Work out the finished part from the listing and answer in its coordinate system (mm). Coordinates: 2 decimals unless noted, no trailing zeros. Write each loop counter-clockwise with the first axis right and the second up, starting at its lowest first coordinate (ties: lowest second). Pieces come first, ordered by that corner, then holes. Notation, with made-up numbers: M 19.5,72.25 L 51.5,72.25 A17 ccw 51.5,88.25 Z; hole C 69.5,69 d10. An arc over 180 degrees is marked long. Answer as CSV lines item,"result". Start each with the question number.
(1) Find the intervals of material crossed by L1, parallel to X at y = 3.15, z = 10.5; L2, parallel to Z at x = 33, y = 2.45, in increasing order. Write a range as [from, to].
(2) A cutting plane is placed at A-A on z = 38.5. Give the vertices of the cut face in (x, y), then the cut area to 3 significant figures.
(3) The mould has two halves that part along X. Classify faces 1 (the flat face through (55, 0, 25)), 2 (the flat face through (78, 3, 27)), 3 (the flat face through (112, 3, 25)): released by +X, released by -X, zero draft, split by the parting line, or undercut.
(4) A cutting plane is placed at B-B on y = 1.25. Count the separate pieces of the cut face and the enclosed holes in it, then the cut area to 3 significant figures.
from build123d import *

# Parameters (mm, degrees)
SKETCH_1_W      = 112
SKETCH_1_H      = 50
SKETCH_1_W_2    = 3
SKETCH_1_H_2    = 20
SKETCH_1_W_3    = 3.2
EXTRUDE_1_DEPTH = 6


with BuildPart() as part:
    # 草图1 → 凸台-拉伸1 (new body)
    with BuildSketch(Plane(origin=(0, 0, 0), x_dir=(1, 0, 0), z_dir=(0, 1, 0))):
        with Locations((56, -25)):
            Rectangle(SKETCH_1_W, SKETCH_1_H)
        with Locations((4.5, -13)):
            Rectangle(SKETCH_1_W_2, SKETCH_1_H_2, mode=Mode.SUBTRACT)
        with Locations((4.5, -37)):
            Rectangle(SKETCH_1_W_2, SKETCH_1_H_2, mode=Mode.SUBTRACT)
        with Locations((107.5, -13)):
            Rectangle(SKETCH_1_W_2, SKETCH_1_H_2, mode=Mode.SUBTRACT)
        with Locations((107.5, -37)):
            Rectangle(SKETCH_1_W_2, SKETCH_1_H_2, mode=Mode.SUBTRACT)
        with Locations((34.4, -37)):
            Rectangle(SKETCH_1_W_3, SKETCH_1_H_2, mode=Mode.SUBTRACT)
        with Locations((34.4, -13)):
            Rectangle(SKETCH_1_W_3, SKETCH_1_H_2, mode=Mode.SUBTRACT)
        with Locations((77.6, -37)):
            Rectangle(SKETCH_1_W_3, SKETCH_1_H_2, mode=Mode.SUBTRACT)
        with Locations((77.6, -13)):
            Rectangle(SKETCH_1_W_3, SKETCH_1_H_2, mode=Mode.SUBTRACT)
    extrude(amount=EXTRUDE_1_DEPTH)


solid = part.part
Here are the results:
1,L1,"x = [0, 3], [6, 32.8], [36, 76], [79.2, 106], [109, 112]"
1,L2,"z = [0, 3], [23, 27], [47, 50]"
2,outline,"M 0,0 L 3,0 L 3,6 L 0,6 Z; M 6,0 L 32.8,0 L 32.8,6 L 6,6 Z; M 36,0 L 76,0 L 76,6 L 36,6 Z; M 79.2,0 L 106,0 L 106,6 L 79.2,6 Z; M 109,0 L 112,0 L 112,6 L 109,6 Z"
2,area,"598 mm^2"
3,face 1,"zero draft"
3,face 2,"undercut"
3,face 3,"released by +X"
4,separate pieces,"1"
4,enclosed holes,"8"
4,area,"5,100 mm^2"
